from build123d import *

# Parameters (mm, degrees)
SKETCH1_W           = 24.7
SKETCH1_H           = 16.55
BOSS_EXTRUDE1_DEPTH = 1.5
SKETCH2_W           = 24.7
SKETCH2_H           = 2.65
CUT_EXTRUDE1_DEPTH  = 0.3


with BuildPart() as part:
    # Sketch1 → Boss-Extrude1 (new body)
    with BuildSketch(Plane(origin=(0, 0, 0), x_dir=(1, 0, 0), z_dir=(0, 1, 0))):
        Rectangle(SKETCH1_W, SKETCH1_H)
    extrude(amount=BOSS_EXTRUDE1_DEPTH)

    # Sketch2 → Cut-Extrude1 (cut)
    with BuildSketch(Plane(origin=(0, 1.5, 0), x_dir=(1, 0, 0), z_dir=(0, 1, 0))):
        with Locations((0, -6.95)):
            Rectangle(SKETCH2_W, SKETCH2_H)
    extrude(amount=-CUT_EXTRUDE1_DEPTH, mode=Mode.SUBTRACT)


solid = part.part
Geometry check sheet. Reference: the model listing, model coordinates, mm. A direction names the side the tool comes from. Coordinates: 2 decimals unless noted, no trailing zeros. Loops run counter-clockwise (first coordinate to the right, second up) from the corner with the lowest first, then second, coordinate; pieces in that order, holes last. Notation, with made-up numbers: (-23.5, -24) - (8.5, -24) arc R15 ccw to (8.5, -4) - close; hole circle Ø6 at (73.5, 30.5). An arc over 180 degrees is marked (long way). Use one line per item in the form item = value. Start each with the question number.
Item 1: Tool access check on faces 1 (the face through (0, 1.5, -1)), 2 (the face through (0, 1.2, 7)). Record the directions out of +Z, -Z, +X, -X, +Y, -Y that give a thin tool (end or side, any length) a straight path to the whole face; none if there is none.
Item 2: Section check A-A, the plane z = 6.75. Enter the section's corners in (x, y), and give its area (3 significant figures).
Item 3: Section check B-B, the plane x = 8.25. Enter the section's corners in (y, z) (3 decimals), and give its area (3 significant figures).
Item 4: Thickness scan on probe 1 along Y at (x, z) = (2.5, 7.25). Record the ranges inside material, lowest first.
Computed:
q1.face_1 = +Z, -Z, +X, -X, +Y
q1.face_2 = +Z, +X, -X, +Y
q2.outline = (-12.35, 0) - (12.35, 0) - (12.35, 1.2) - (-12.35, 1.2) - close
q2.area = 29.6 mm2
q3.outline = (0, -8.275) - (1.5, -8.275) - (1.5, 5.625) - (1.2, 5.625) - (1.2, 8.275) - (0, 8.275) - close
q3.area = 24.0 mm2
q4.probe_1 = 0 to 1.2
